```python
from build123d import *

# Parameters (mm, degrees)
F0_R     = 1.6
F0_W     = 48
F0_H     = 5
F0_W_2   = 45
F0_H_2   = 9
F3_DEPTH = 5
F1_R     = 1.6
F2_R     = 2.5
F4_DEPTH = 5


with BuildPart() as f3:
    # F0 (on Front) → F3 (new body)
    with BuildSketch(Plane.XZ):
        Polygon((-145, -62.300583), (145, -62.300583), (145, -39.300583), (150, -39.300583), (150, -16.300583), (145, -16.300583), (145, 6.699417), (150, 6.699417), (150, 29.699417), (145, 29.699417), (145, 52.699417), (145, 57.699417), (120, 57.699417), (120, 52.699417), (-120, 52.699417), (-120, 57.699417), (-145, 57.699417), (-145, 52.699417), (-145, 29.699417), (-150, 29.699417), (-150, 6.699417), (-145, 6.699417), (-145, -16.300583), (-150, -16.300583), (-150, -39.300583), (-145, -39.300583), align=None)
        with Locations((-108, -51.800583)):
            Circle(F0_R, mode=Mode.SUBTRACT)
        with Locations((-102, -51.800583)):
            Circle(F0_R, mode=Mode.SUBTRACT)
        with Locations((-3, -51.800583)):
            Circle(F0_R, mode=Mode.SUBTRACT)
        with Locations((-96, -14.800583)):
            Rectangle(F0_W, F0_H, mode=Mode.SUBTRACT)
        with Locations((-92.5, -2.800583)):
            Rectangle(F0_W_2, F0_H_2, mode=Mode.SUBTRACT)
        with Locations((3, -51.800583)):
            Circle(F0_R, mode=Mode.SUBTRACT)
        with Locations((102, -51.800583)):
            Circle(F0_R, mode=Mode.SUBTRACT)
        with Locations((108, -51.800583)):
            Circle(F0_R, mode=Mode.SUBTRACT)
        with Locations((0, -14.800583)):
            Rectangle(F0_W, F0_H, mode=Mode.SUBTRACT)
        with Locations((96, -14.800583)):
            Rectangle(F0_W, F0_H, mode=Mode.SUBTRACT)
        with Locations((-108, 47.199417)):
            Circle(F0_R, mode=Mode.SUBTRACT)
        with Locations((-102, 47.199417)):
            Circle(F0_R, mode=Mode.SUBTRACT)
        with Locations((-3, 47.199417)):
            Circle(F0_R, mode=Mode.SUBTRACT)
        with Locations((3, 47.199417)):
            Circle(F0_R, mode=Mode.SUBTRACT)
        with Locations((102, 47.199417)):
            Circle(F0_R, mode=Mode.SUBTRACT)
        with Locations((108, 47.199417)):
            Circle(F0_R, mode=Mode.SUBTRACT)
    extrude(amount=F3_DEPTH)

    # F1 (on face) + F2 (on face) → F4 (cut)
    with BuildSketch(Plane.XZ):
        with Locations((-138.5, 28.199417)):
            Circle(F1_R)
        with Locations((-138.5, 9.199417)):
            Circle(F1_R)
        with Locations((-40.5, 9.199417)):
            Circle(F1_R)
        with Locations((-40.5, 28.199417)):
            Circle(F1_R)
    with BuildSketch(Plane.XZ):
        with Locations((135, 37.199417)):
            Circle(F2_R)
        with Locations((135, 27.199417)):
            Circle(F2_R)
        with Locations((135, 17.199417)):
            Circle(F2_R)
        with Locations((135, 7.199417)):
            Circle(F2_R)
        with Locations((125, 37.199417)):
            Circle(F2_R)
        with Locations((125, 27.199417)):
            Circle(F2_R)
        with Locations((125, 17.199417)):
            Circle(F2_R)
        with Locations((125, 7.199417)):
            Circle(F2_R)
        with Locations((115, 37.199417)):
            Circle(F2_R)
        with Locations((115, 27.199417)):
            Circle(F2_R)
        with Locations((115, 17.199417)):
            Circle(F2_R)
        with Locations((115, 7.199417)):
            Circle(F2_R)
        with Locations((105, 37.199417)):
            Circle(F2_R)
        with Locations((105, 27.199417)):
            Circle(F2_R)
        with Locations((105, 17.199417)):
            Circle(F2_R)
        with Locations((105, 7.199417)):
            Circle(F2_R)
        with Locations((95, 37.199417)):
            Circle(F2_R)
        with Locations((95, 27.199417)):
            Circle(F2_R)
        with Locations((95, 17.199417)):
            Circle(F2_R)
        with Locations((95, 7.199417)):
            Circle(F2_R)
        with Locations((85, 37.199417)):
            Circle(F2_R)
        with Locations((85, 27.199417)):
            Circle(F2_R)
        with Locations((85, 17.199417)):
            Circle(F2_R)
        with Locations((85, 7.199417)):
            Circle(F2_R)
        with Locations((75, 37.199417)):
            Circle(F2_R)
        with Locations((75, 27.199417)):
            Circle(F2_R)
        with Locations((75, 17.199417)):
            Circle(F2_R)
        with Locations((75, 7.199417)):
            Circle(F2_R)
        with Locations((65, 37.199417)):
            Circle(F2_R)
        with Locations((65, 27.199417)):
            Circle(F2_R)
        with Locations((65, 17.199417)):
            Circle(F2_R)
        with Locations((65, 7.199417)):
            Circle(F2_R)
        with Locations((55, 37.199417)):
            Circle(F2_R)
        with Locations((55, 27.199417)):
            Circle(F2_R)
        with Locations((55, 17.199417)):
            Circle(F2_R)
        with Locations((55, 7.199417)):
            Circle(F2_R)
        with Locations((-135, -42.300583)):
            Circle(F2_R)
        with Locations((-135, -32.300583)):
            Circle(F2_R)
        with Locations((-125, -42.300583)):
            Circle(F2_R)
        with Locations((-125, -32.300583)):
            Circle(F2_R)
        with Locations((-115, -42.300583)):
            Circle(F2_R)
        with Locations((-115, -32.300583)):
            Circle(F2_R)
        with Locations((-105, -42.300583)):
            Circle(F2_R)
        with Locations((-105, -32.300583)):
            Circle(F2_R)
        with Locations((-95, -42.300583)):
            Circle(F2_R)
        with Locations((-95, -32.300583)):
            Circle(F2_R)
        with Locations((-85, -42.300583)):
            Circle(F2_R)
        with Locations((-85, -32.300583)):
            Circle(F2_R)
        with Locations((-75, -42.300583)):
            Circle(F2_R)
        with Locations((-75, -32.300583)):
            Circle(F2_R)
        with Locations((-65, -42.300583)):
            Circle(F2_R)
        with Locations((-65, -32.300583)):
            Circle(F2_R)
        with Locations((-55, -42.300583)):
            Circle(F2_R)
        with Locations((-55, -32.300583)):
            Circle(F2_R)
        with Locations((-45, -42.300583)):
            Circle(F2_R)
        with Locations((-45, -32.300583)):
            Circle(F2_R)
        with Locations((-35, -42.300583)):
            Circle(F2_R)
        with Locations((-35, -32.300583)):
            Circle(F2_R)
        with Locations((-25, -42.300583)):
            Circle(F2_R)
        with Locations((-25, -32.300583)):
            Circle(F2_R)
        with Locations((-15, -42.300583)):
            Circle(F2_R)
        with Locations((-15, -32.300583)):
            Circle(F2_R)
        with Locations((-5, -42.300583)):
            Circle(F2_R)
        with Locations((-5, -32.300583)):
            Circle(F2_R)
        with Locations((5, -42.300583)):
            Circle(F2_R)
        with Locations((5, -32.300583)):
            Circle(F2_R)
        with Locations((15, -42.300583)):
            Circle(F2_R)
        with Locations((15, -32.300583)):
            Circle(F2_R)
        with Locations((25, -42.300583)):
            Circle(F2_R)
        with Locations((25, -32.300583)):
            Circle(F2_R)
        with Locations((35, -42.300583)):
            Circle(F2_R)
        with Locations((35, -32.300583)):
            Circle(F2_R)
        with Locations((45, -42.300583)):
            Circle(F2_R)
        with Locations((45, -32.300583)):
            Circle(F2_R)
        with Locations((55, -42.300583)):
            Circle(F2_R)
        with Locations((55, -32.300583)):
            Circle(F2_R)
    extrude(amount=F4_DEPTH, mode=Mode.SUBTRACT)


solid = f3.part
```
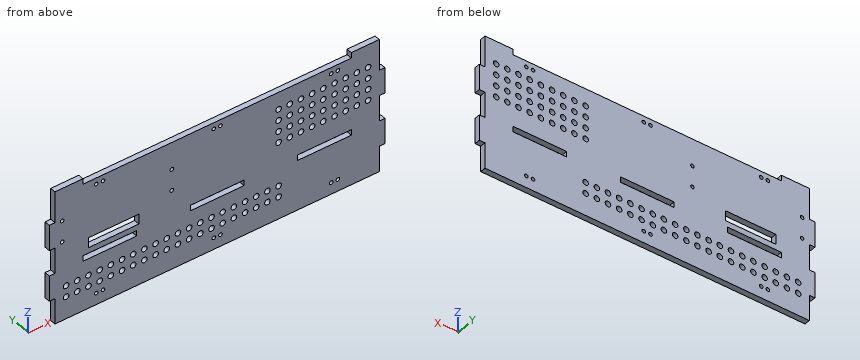
For this review, take the finished solid that the model builds, in its own axes (mm). Round coordinates to 2 decimals unless told otherwise and drop trailing zeros.
Q1. Insertion check: P1, Ø3, axis at y = -1.5, z = 32.5, coming from the -X side; P2, Ø4.5, axis at x = -15, z = -32.3, coming from the +Y side; P3, Ø1.5, axis at y = -3.5, z = 55, coming from the +X side. Each pin has a flat end and moves straight along its axis. Give the tip position at first contact, or say it passes through.
Findings below:
P1: stops at x = -145
P2: passes through
P3: stops at x = 145
Q2. Wall thickness on line 1 (Z direction, x = 115, y = -2.2); line 2 (Z direction, x = -108, y = -3.15); line 3 (Z direction, x = 5, y = -2.55): over which ranges is each line inside the solid? List them lowest first.
Findings below:
line 1: z = -62.3 to -17.3, -12.3 to 4.7, 9.7 to 14.7, 19.7 to 24.7, 29.7 to 34.7, 39.7 to 52.7
line 2: z = -62.3 to -53.4, -50.2 to -17.3, -12.3 to -7.3, 1.7 to 45.6, 48.8 to 52.7
line 3: z = -62.3 to -44.8, -39.8 to -34.8, -29.8 to -17.3, -12.3 to 52.7
Q3. We need section A-A, the plane y = -3.95. State how many separate pieces and enclosed holes the cut face has, plus the area to 3 significant figures.
Findings below:
separate pieces: 1
enclosed holes: 96
area: 31,300 mm2
